Part print with two shaded views. Sizes in mm from the minimum x, y, z corner. A direction names the side the tool comes from. Round coordinates to 2 decimals unless told otherwise and drop trailing zeros. Loops run counter-clockwise (first coordinate to the right, second up) from the corner with the lowest first, then second, coordinate; pieces in that order, holes last. Notation, with made-up numbers: (51, 74.25) -> (82, 74.25) arc R15 ccw to (82, 88.25) -> close; hole circle Ø7 at (-22, -29). An arc over 180 degrees is marked (long way). Use a Markdown table: item, result. Add a question column.
Item 1: Cut at B-B, the plane x = 245.5. List the corners of the cut face in (y, z).
Item 2: Which spindle directions (+Z, -Z, +X, -X, +Y, -Y) get a long thin tool onto all of the face, cutting with end or side? Do the marked faces 4 and 5. Say none if no direction does.
Item 3: Cut at C-C, the plane y = 60.5. List the corners of the cut face in (x, z).
Item 4: Cut at A-A, the plane z = 438. List the corners of the cut face in (x, y).
Item 5: Flat gauge pin, fed straight in: pin 1 (6 mm diameter, centred on x = 466, y = 323, fed in from +Z). Where does the tip first touch, or does it go through?
Item 6: Two-plate mould, pull along X, no slides. Class the marked faces 1, 2 and 3: pulls with the +X half, pulls with the -X half, needs draft (parallel to the pull), parting line crosses it, or undercut.
Item 7: Probe line 1 (Z direction, x = 294.5, y = 368.5); line 2 (X direction, y = 181, z = 115); line 3 (Z direction, x = 50.5, y = 279) (1 decimal). List the from-to ranges inside material, lowest first. Write a range as [from, to].
Item 8: Cut at D-D, the plane x = 341.5. List the corners of the cut face in (y, z), plus the area to 3 significant figures.
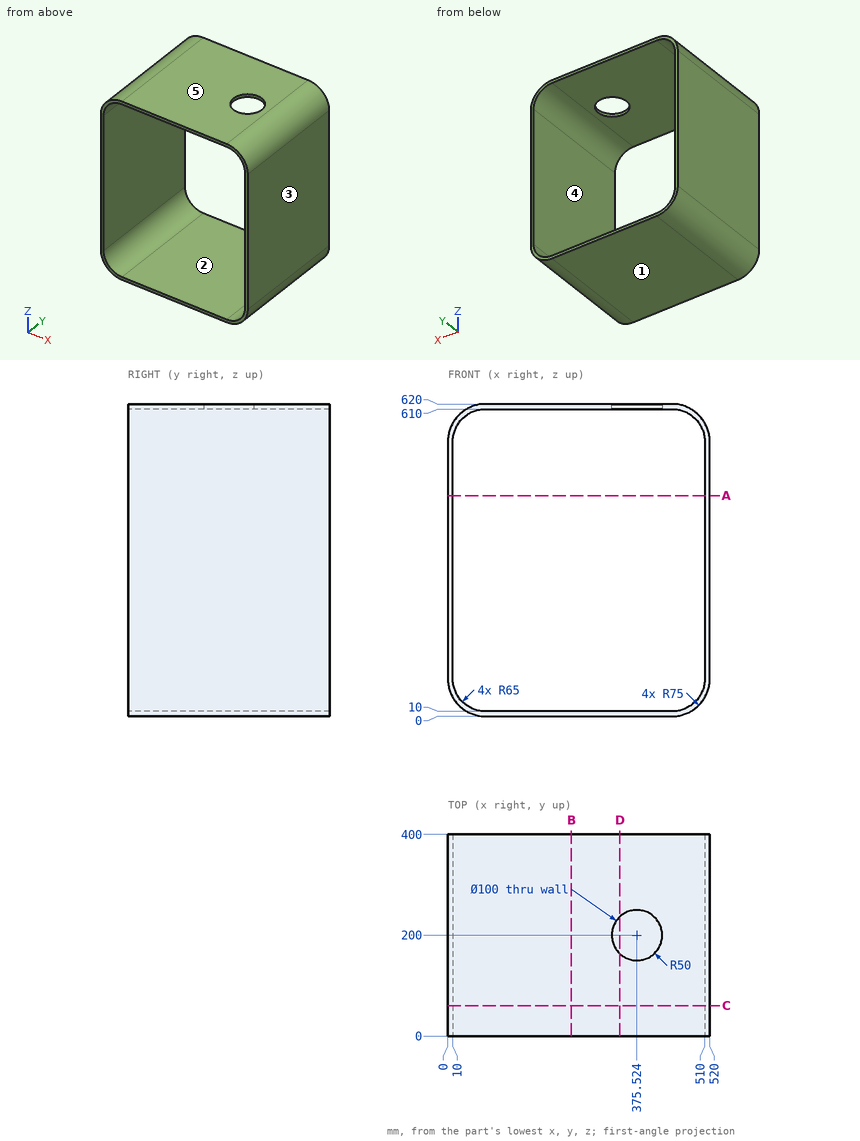
A:
| question | item | result |
|---|---|---|
| 1 | outline | (0, 0) -> (400, 0) -> (400, 10) -> (0, 10) -> close; (0, 610) -> (400, 610) -> (400, 620) -> (0, 620) -> close |
| 2 | face 4 | +Y, -Y |
| 2 | face 5 | +Z, +X, -X, +Y, -Y |
| 3 | outline | (0, 75) arc R75 ccw to (75, 0) -> (445, 0) arc R75 ccw to (520, 75) -> (520, 545) arc R75 ccw to (445, 620) -> (75, 620) arc R75 ccw to (0, 545) -> close; hole (10, 75) arc R65 ccw to (75, 10) -> (445, 10) arc R65 ccw to (510, 75) -> (510, 545) arc R65 ccw to (445, 610) -> (75, 610) arc R65 ccw to (10, 545) -> close |
| 4 | outline | (0, 0) -> (10, 0) -> (10, 400) -> (0, 400) -> close; (510, 0) -> (520, 0) -> (520, 400) -> (510, 400) -> close |
| 5 | pin 1 | stops at z = 617.81 |
| 6 | face 1 | needs draft |
| 6 | face 2 | undercut |
| 6 | face 3 | pulls with the +X half |
| 7 | line 1 | z = [0, 10], [610, 620] |
| 7 | line 2 | x = [0, 10], [510, 520] |
| 7 | line 3 | z = [4.1, 14.8], [605.2, 615.9] |
| 8 | outline | (0, 0) -> (400, 0) -> (400, 10) -> (0, 10) -> close; (0, 610) -> (163.36, 610) -> (163.36, 620) -> (0, 620) -> close; (236.64, 610) -> (400, 610) -> (400, 620) -> (236.64, 620) -> close |
| 8 | area | 7,270 mm^2 |
